Could you check a few things on this model? Use its own coordinates, in mm. A direction names the side the tool comes from. Round coordinates to 2 decimals unless told otherwise and drop trailing zeros. Loops run counter-clockwise (first coordinate to the right, second up) from the corner with the lowest first, then second, coordinate; pieces in that order, holes last. Notation, with made-up numbers: M 79.25,51.25 L 92.25,51.25 A11 ccw 92.25,65.25 Z; hole C -31.75,10.25 d4. An arc over 180 degrees is marked long. Answer in a Markdown table with one row per item.
Autodesk Inventor part; units mm, degrees
ref_plane "YZ Plane" through (0, 0, 0) normal (1, 0, 0) x (0, 1, 0)
ref_plane "XZ Plane" through (0, 0, 0) normal (0, 1, 0) x (-1, 0, 0)
ref_plane "XY Plane" through (0, 0, 0) normal (0, 0, 1) x (1, 0, 0)
sketch "Sketch1" plane through (0, 0, 0) normal (0, 0, 1) x (1, 0, 0)
  line L0 (0, 0) -> (25.4, 0)
  line L1 (-6.35, 6.35) -> (0, 0)
  line L2 (31.75, 6.35) -> (25.4, 0)
  line L3 (-6.35, 6.35) -> (-6.35, 25.4)
  line L4 (-6.35, 25.4) -> (0, 31.75)
  line L5 (0, 31.75) -> (25.4, 31.75)
  line L6 (25.4, 31.75) -> (31.75, 25.4)
  line L7 (31.75, 25.4) -> (31.75, 22.225)
  line L8 (31.75, 22.225) -> (19.05, 22.225)
  line L9 (19.05, 26.67) -> (19.05, 22.225)
  line L10 (1.27, 19.05) -> (1.27, 9.525)
  line L11 (4.445, 6.35) -> (1.27, 9.525)
  line L12 (1.27, 19.05) -> (1.27, 23.495)
  line L13 (4.445, 26.67) -> (1.27, 23.495)
  line L14 (31.75, 6.35) -> (31.75, 9.525)
  line L15 (31.75, 9.525) -> (19.05, 9.525)
  line L16 (19.05, 9.525) -> (19.05, 6.35)
  line L17 (19.05, 6.35) -> (4.445, 6.35)
  line L18 (4.445, 26.67) -> (19.05, 26.67)
  dimension "d0" = 25.4
  dimension "d6" = 19.05
  dimension "d7" = 25.4
  dimension "d8" = 3.175
  dimension "d9" = 12.7
  dimension "d21" = 3.175
  dimension "d22" = 12.7
  dimension "d23" = 3.175
extrude "Extrusion1" add sketch "Sketch1" along normal blind 6.35
properties part number "Assignment 2.1 - C-Clip"
1) I want a section at B-B, the plane z = 5. Please give me the cut outline in (x, y) (3 decimals).
Computed:
| item | result |
|---|---|
| outline | M -6.35,6.35 L 0,0 L 25.4,0 L 31.75,6.35 L 31.75,9.525 L 19.05,9.525 L 19.05,6.35 L 4.445,6.35 L 1.27,9.525 L 1.27,23.495 L 4.445,26.67 L 19.05,26.67 L 19.05,22.225 L 31.75,22.225 L 31.75,25.4 L 25.4,31.75 L 0,31.75 L -6.35,25.4 Z |
2) If we mould it in two halves opening along X, with no side actions, what happens to faces 1 (the face through (31.75, 8, 3)), 2 (the face through (19.05, 24, 3)), 3 (the face through (25, 9.525, 3)), 4 (the face through (19.05, 8, 3))? For each: released by +X, released by -X, zero draft, split by the parting line, or undercut.
Computed:
| item | result |
|---|---|
| face 1 | released by +X |
| face 2 | undercut |
| face 3 | zero draft |
| face 4 | undercut |
3) Which directions (+Z, -Z, +X, -X, +Y, -Y) give clear straight access to the entire face, cutting with the end or side of a thin tool? Please do faces 5 (the face through (28.6, 3.2, 3.1)), 6 (the face through (2.88, 7.915, 3.131)), 7 (the face through (25, 22.225, 3)).
Computed:
| item | result |
|---|---|
| face 5 | +Z, -Z, +X, -Y |
| face 6 | +Z, -Z |
| face 7 | +Z, -Z, +X |
4) I want a section at D-D, the plane x = -4. Please give me the cut outline in (y, z), plus the area to 3 significant figures.
Computed:
| item | result |
|---|---|
| outline | M 4,0 L 27.75,0 L 27.75,6.35 L 4,6.35 Z |
| area | 151 mm² |
5) I need wall thicknesses on line 1 (Y direction, x = 7, z = 5.75); line 2 (X direction, y = 22.5, z = 1); line 3 (Y direction, x = 26.5, z = 3.25) (3 decimals). Which ranges of each line are inside material? Lowest first, please.
Computed:
| item | result |
|---|---|
| line 1 | y = 0 to 6.35, 26.67 to 31.75 |
| line 2 | x = -6.35 to 1.27, 19.05 to 31.75 |
| line 3 | y = 1.1 to 9.525, 22.225 to 30.65 |
6) I want a section at C-C, the plane y = 9. Please give me the cut outline in (x, z) (3 decimals).
Computed:
| item | result |
|---|---|
| outline | M -6.35,0 L 1.795,0 L 1.795,6.35 L -6.35,6.35 Z; M 19.05,0 L 31.75,0 L 31.75,6.35 L 19.05,6.35 Z |
7) I want a section at A-A, the plane x = 10.5. Please give me the cut outline in (y, z).
Computed:
| item | result |
|---|---|
| outline | M 0,0 L 6.35,0 L 6.35,6.35 L 0,6.35 Z; M 26.67,0 L 31.75,0 L 31.75,6.35 L 26.67,6.35 Z |
8) Will these pins go through, and if not, where does the flat tip stop? P1, Ø1.5, axis at y = 27.5, z = 2.5, coming from the -X side; P2, Ø1.9, axis at x = 27, z = 2.5, coming from the +Y side.
Computed:
| item | result |
|---|---|
| P1 | stops at x = -5 |
| P2 | stops at y = 31.1 |
